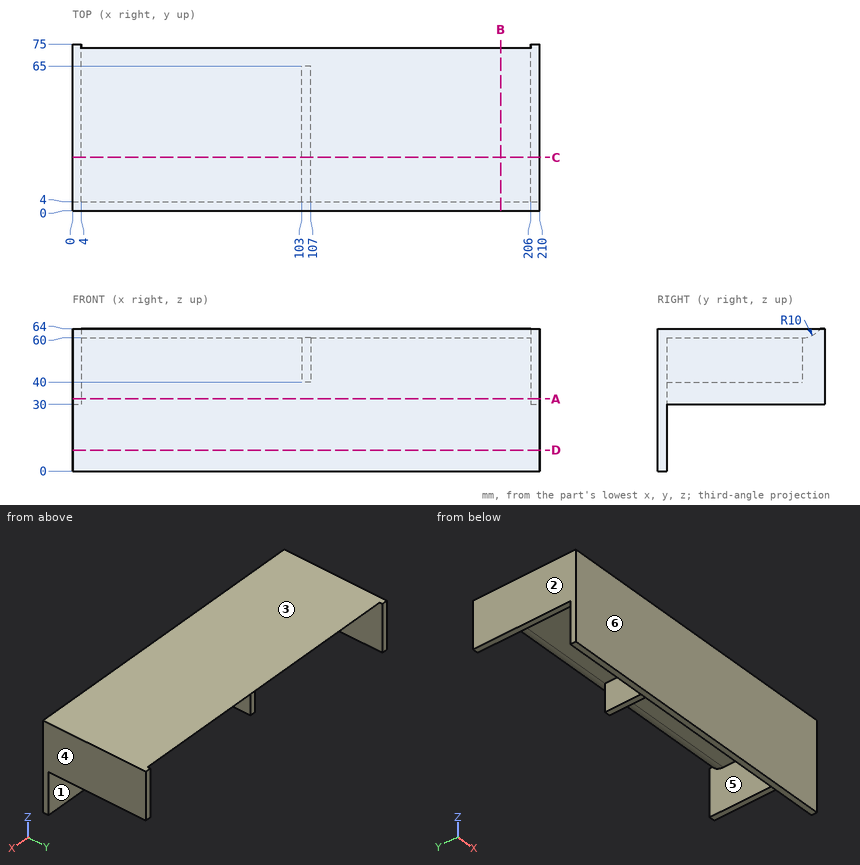
Verification items for this drawing (mm, ordinates from the low corner). A direction names the side the tool comes from. Give positions to 0.01 mm unless a question says otherwise; leave off trailing zeros. Loops run counter-clockwise (first coordinate to the right, second up) from the corner with the lowest first, then second, coordinate; pieces in that order, holes last. Notation, with made-up numbers: M -18,-35.5 L -11,-35.5 A22 cw -11,-23.5 Z; hole C 38.25,82 d1. An arc over 180 degrees is marked long. Answer as a JSON object with one key per item and string values. Group by question number.
Q1. Cross-section at B-B on x = 192.5. Record the cut outline in (y, z).
Q2. Material ranges on line 1 along X through (y, z) = (36, 42); line 2 along X through (y, z) = (69.5, 60); line 3 along Z through (x, y) = (187, 23.5), recorded low to high. Write a range as [from, to].
Q3. Access from +Z, -Z, +X, -X, +Y, -Y to the whole of each face (thin tool, end or side, straight path). Record for the marked faces 5 and 6.
Q4. Release check for a two-part mould opening along X. For the marked faces 1, 2, 3 and 4 record: released by +X, released by -X, zero draft, split by the parting line, or undercut.
Q5. Cross-section at A-A on z = 32.5. Record the cut outline in (x, y), then the cut area to 3 significant figures.
Q6. Go/stop test with flat-tipped pins: P1, Ø1.2, axis at x = 106, y = 23, coming from the -Z side; P2, Ø3, axis at x = 2, y = 42.5, coming from the -Z side; P3, Ø1.5, axis at x = 111, z = 52, coming from the +Y side. Record where each tip stops, or that it passes through.
Q7. Cross-section at C-C on y = 24. Record the cut outline in (x, z), then the cut area to 3 significant figures.
Q8. Cross-section at D-D on z = 9.5. Record the cut outline in (x, y).
Evaluation:
{
 "1": {"outline": "M 0,0 L 4,0 L 4,60 L 65,60 A10 ccw 73,64 L 0,64 Z"},
 "2": {"line 1": "x = [0, 4], [103, 107], [206, 210]", "line 2": "x = [0, 4], [206, 210]", "line 3": "z = [60, 64]"},
 "3": {"face 5": "-Z, +Y", "face 6": "+Z, -Z, +X, -X, -Y"},
 "4": {"face 1": "undercut", "face 2": "released by -X", "face 3": "zero draft", "face 4": "released by +X"},
 "5": {"outline": "M 0,0 L 210,0 L 210,75 L 206,75 L 206,4 L 4,4 L 4,75 L 0,75 Z", "area": "1,410 mm2"},
 "6": {"P1": "stops at z = 40", "P2": "stops at z = 30", "P3": "stops at y = 4"},
 "7": {"outline": "M 0,30 L 4,30 L 4,60 L 103,60 L 103,40 L 107,40 L 107,60 L 206,60 L 206,30 L 210,30 L 210,64 L 0,64 Z", "area": "1,160 mm2"},
 "8": {"outline": "M 0,0 L 210,0 L 210,4 L 0,4 Z"}
}
